For this review, use the dimensioned drawing (mm, ordinates from the lowest corner) and the shaded views. A direction names the side the tool comes from. Coordinates: 2 decimals unless noted, no trailing zeros. Loops run counter-clockwise (first coordinate to the right, second up) from the corner with the lowest first, then second, coordinate; pieces in that order, holes last. Notation, with made-up numbers: M -36.75,12.25 L -0.75,12.25 A31 cw -0.75,49.25 Z; hole C 34,15.25 d11. An arc over 180 degrees is marked long. Write item = value, one per line. Start each with the question number.
Q1. We need section A-A on x = 16.86. Give the boundary of the cut face in (y, z), and give its area (3 significant figures).
Q2. For the marked faces 1 and 2, list the 3-axis set-ups (+Z, -Z, +X, -X, +Y, -Y) from which the entire face can be reached by the end or side of a thin tool; tool diameter is ignored.
Q3. Mouldability with a two-part tool opening along X and no side actions: class the marked faces 3, 4, 5 and 6 as released by +X, released by -X, zero draft, split by the parting line, or undercut.
Q4. We need section C-C on x = 9. Give the boundary of the cut face in (y, z).
Q5. We need section B-B on y = 4.5. Give the boundary of the cut face in (x, z) (1 decimal).
Q6. Wall thickness on probe 1 along Y at (x, z) = (16.86, 1.6); probe 2 along Y at (x, z) = (8, 2.6); probe 3 along Y at (x, z) = (18, 0.6) (1 decimal): over which ranges is each line inside the solid? List them lowest first.
Q7. We need section D-D on z = 3.75. Give the boundary of the cut face in (x, y) (1 decimal), and give its area (3 significant figures).
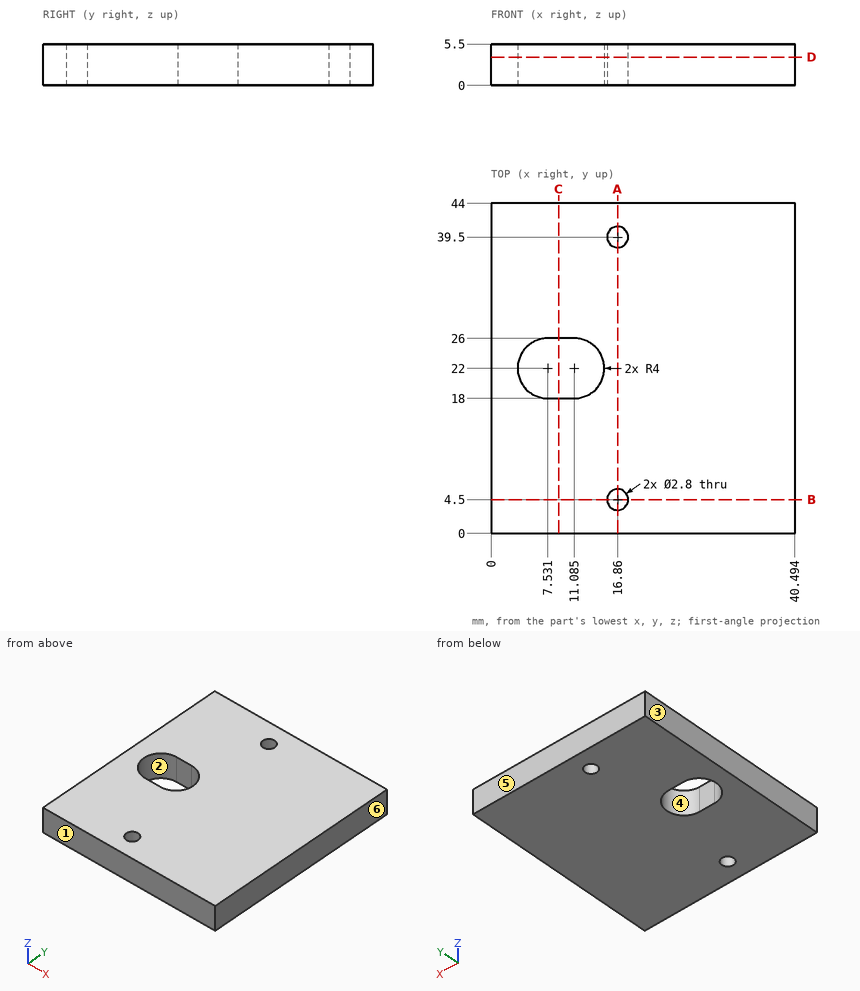
Returned:
q1.outline = M 0,0 L 3.1,0 L 3.1,5.5 L 0,5.5 Z; M 5.9,0 L 38.1,0 L 38.1,5.5 L 5.9,5.5 Z; M 40.9,0 L 44,0 L 44,5.5 L 40.9,5.5 Z
q1.area = 211 mm^2
q2.face_1 = +Z, -Z, +X, -X, -Y
q2.face_2 = +Z, -Z
q3.face_3 = released by -X
q3.face_4 = undercut
q3.face_5 = zero draft
q3.face_6 = released by +X
q4.outline = M 0,0 L 18,0 L 18,5.5 L 0,5.5 Z; M 26,0 L 44,0 L 44,5.5 L 26,5.5 Z
q5.outline = M 0,0 L 15.5,0 L 15.5,5.5 L 0,5.5 Z; M 18.3,0 L 40.5,0 L 40.5,5.5 L 18.3,5.5 Z
q6.probe_1 = 0 to 3.1, 5.9 to 38.1, 40.9 to 44
q6.probe_2 = 0 to 18, 26 to 44
q6.probe_3 = 0 to 3.7, 5.3 to 38.7, 40.3 to 44
q7.outline = M 0,0 L 40.5,0 L 40.5,44 L 0,44 Z; hole M 7.5,18 L 11.1,18 A4 ccw 11.1,26 L 7.5,26 A4 ccw Z; hole C 16.9,4.5 d2.8; hole C 16.9,39.5 d2.8
q7.area = 1,690 mm^2
